The model under review builds one solid part; all positions refer to its coordinate system, in mm. A direction names the side the tool comes from. Coordinates: 2 decimals unless noted, no trailing zeros. Loops run counter-clockwise (first coordinate to the right, second up) from the corner with the lowest first, then second, coordinate; pieces in that order, holes last. Notation, with made-up numbers: (77, -14) -> (129, -14) arc R24 cw to (129, 14) -> close; hole circle Ø9 at (-25, 59). An arc over 180 degrees is marked (long way). One line per question, with ' | ' between items. Start each with the question number.
from build123d import *

# Parameters (mm, degrees)
F1_DEPTH = 100
F2_SIZE2 = 15
F2_SIZE  = 15
F3_W     = 208
F3_H     = 8.5
F4_DEPTH = 2


with BuildPart() as f1:
    # F0 (on Front) → F1 (new body)
    with BuildSketch(Plane.XZ):
        Polygon((7, 0), (0, 0), (0, -17), (208, -17), (208, 0), (201, 0), (201, -11), (191.25, -11), (191.25, 0), (184.25, 0), (184.25, -11), (174.5, -11), (174.5, 0), (167.5, 0), (167.5, -11), (157.75, -11), (157.75, 0), (150.75, 0), (150.75, -11), (141, -11), (141, 0), (134, 0), (134, -11), (124.25, -11), (124.25, 0), (117.25, 0), (117.25, -11), (107.5, -11), (107.5, 0), (100.5, 0), (100.5, -11), (90.75, -11), (90.75, 0), (83.75, 0), (83.75, -11), (74, -11), (74, 0), (67, 0), (67, -11), (57.25, -11), (57.25, 0), (50.25, 0), (50.25, -11), (40.5, -11), (40.5, 0), (33.5, 0), (33.5, -11), (23.75, -11), (23.75, 0), (16.75, 0), (16.75, -11), (7, -11), align=None)
    extrude(amount=F1_DEPTH)

    # F2
    f2_edges = [f1.edges().sort_by_distance(p)[0] for p in [
        (0, 0, -8.5),
    ]]
    chamfer(f2_edges, length=F2_SIZE, length2=F2_SIZE2)

    # F3 (on face) → F4 (join)
    with BuildSketch(Plane.XZ.offset(100)):
        with Locations((104, -12.75)):
            Rectangle(F3_W, F3_H)
    extrude(amount=F4_DEPTH)


solid = f1.part
1) Wall thickness on L1, parallel to Z at x = 115, y = -7.5; L2, parallel to Y at x = 74.5, z = -10.5; L3, parallel to Y at x = 18, z = -4.5: over which ranges is each line inside the solid? List them lowest first.
2) Consider section A-A, the plane x = 179. Write out the cut boundary in (y, z).
3) Insertion check: pin 1 Ø3.5 at (x, z) = (136.5, -5) entering from -Y; pin 2 Ø6 at (x, z) = (42.5, -2) entering from +Y; pin 3 Ø8 at (x, y) = (112, -74) entering from +Z; pin 4 Ø1.2 at (x, z) = (13, -9.5) entering from +Y. Each pin has a flat end and moves straight along its axis. Give the tip position at first contact, or say it passes through.
4) Mouldability with a two-part tool opening along X and no side actions: class faces 4 (the face through (188, -100, -4)), 5 (the face through (146, -49, -11)), 6 (the face through (0, -58, -9)) as +X half, -X half, draft (parallel to the pull), parting line (faces both ways), or undercut.
5) Consider section B-B, the plane z = -5.25. Give the number of separate pieces and of enclosed holes in the cut face, plus the area to 3 significant figures.
6) Machinability: for faces 1 (the face through (191.25, -49, -6)), 2 (the face through (188, -49, 0)), 3 (the face through (37, -100, -4)), which of the approach directions +Z, -Z, +X, -X, +Y, -Y give a long, thin tool a straight path to every point of the face, cutting with its end or side? Answer none if there is none.
Filled sheet:
1) L1: -17 to -11 | L2: -102 to -100 | L3: -100 to 0
2) outline: (-102, -17) -> (0, -17) -> (0, -11) -> (-100, -11) -> (-100, -8.5) -> (-102, -8.5) -> close
3) pin 1: y = -100 | pin 2: y = 0 | pin 3: z = -11 | pin 4: y = -100
4) face 4: draft | face 5: undercut | face 6: -X half
5) separate pieces: 13 | enclosed holes: 0 | area: 9,020 mm^2
6) face 1: +Z, +Y | face 2: +Z, +X, -X, +Y, -Y | face 3: +Z, +X, -X, -Y
